from build123d import *

# Parameters (mm, degrees)
BOSS_EXTRUDE1_DEPTH = 24
SKETCH3_R           = 1.9
SKETCH3_R_2         = 0.9
BOSS_EXTRUDE2_DEPTH = 1
SKETCH4_R           = 1.15
CUT_EXTRUDE2_DEPTH  = 4
CUT_EXTRUDE3_DEPTH  = 30


with BuildPart() as part:
    # Sketch1 → Boss-Extrude1 (new body)
    with BuildSketch(Plane(origin=(0, 0, 0), x_dir=(1, 0, 0), z_dir=(0, 1, 0))):
        Polygon((0.758759529, 5.315), (5, 5.315), (5, -7.215), (1.398203198, -7.215), (-1.03, -7.215), (-1.03, -1.785), (4, -1.785), (4, -0.115), (-1.03, -0.115), (-1.03, 5.315), align=None)
    extrude(amount=BOSS_EXTRUDE1_DEPTH)

    # Sketch3 → Boss-Extrude2 (add)
    with BuildSketch(Plane(origin=(5, 0, 0), x_dir=(0, 0, -1), z_dir=(1, 0, 0))):
        with Locations((2.815, 19)):
            Circle(SKETCH3_R)
        with Locations((2.815, 19)):
            Circle(SKETCH3_R_2, mode=Mode.SUBTRACT)
        with Locations((2.815, 5)):
            Circle(SKETCH3_R)
        with Locations((2.815, 5)):
            Circle(SKETCH3_R_2, mode=Mode.SUBTRACT)
    extrude(amount=BOSS_EXTRUDE2_DEPTH)

    # Sketch4 → Cut-Extrude2 (cut)
    with BuildSketch(Plane(origin=(5, 0, 0), x_dir=(0, 0, -1), z_dir=(1, 0, 0))):
        with Locations((2.815, 19)):
            Circle(SKETCH4_R)
        with Locations((2.815, 5)):
            Circle(SKETCH4_R)
    extrude(amount=-CUT_EXTRUDE2_DEPTH, mode=Mode.SUBTRACT)

    # Sketch6 → Cut-Extrude3 (cut)
    with BuildSketch(Plane(origin=(0, 24, 0), x_dir=(1, 0, 0), z_dir=(0, 1, 0))):
        Polygon((-1.03, -0.115), (4, -0.115), (-1.03, 1.385), align=None)
        Polygon((4, -1.785), (-1.03, -1.785), (-1.03, -3.285), align=None)
    extrude(amount=-CUT_EXTRUDE3_DEPTH, mode=Mode.SUBTRACT)


solid = part.part
For this review, take the finished solid that the model builds, in its own axes (mm). A direction names the side the tool comes from. Give positions to 0.01 mm unless a question says otherwise; leave off trailing zeros. Loops run counter-clockwise (first coordinate to the right, second up) from the corner with the lowest first, then second, coordinate; pieces in that order, holes last.
Item 1: For line 1 along X through (y, z) = (18.5, -2); line 2 along Z through (x, y) = (3, 19.5) (3 decimals); line 3 along Y through (x, z) = (4.5, -3.75), list the stretches that pass through material, from the lowest coordinate up.
Item 2: Take a section at B-B, the plane x = 3.25. State the section outline as (y, z) points (3 decimals), and give its area (3 significant figures).
Item 3: Take a section at C-C, the plane z = -2.25. State the section outline as (x, y) points.
Item 4: Tool access review of faces 1 (the cylindrical face through (5.493, 20.884, -2.568)), 2 (the cylindrical face through (3.03, 6.14, -2.67)), 3 (the flat face through (2, 12, -5.315)), 4 (the flat face through (1.45, 12.168, 2.545)): name each direction out of +Z, -Z, +X, -X, +Y, -Y from which nothing blocks a thin tool from reaching the whole face with its end or side.
Item 5: Take a section at A-A, the plane y = 5. State the section outline as (x, z) points (3 decimals), and give its area (3 significant figures).
Item 6: Take a section at D-D, the plane x = 0.5. State the section outline as (y, z) points (3 decimals).
Item 7: Insertion check: pin 1 (1.5 mm diameter, centred on y = 14, z = -3.5, fed in from +X); pin 2 (1.6 mm diameter, centred on y = 19, z = -2.815, fed in from +X). Each pin has a flat end and moves straight along its axis. Give the tip position at first contact, or say it passes through.
Item 8: Draft analysis for pull direction Z (two halves, no side actions). For faces 5 (the cylindrical face through (5.493, 19.892, -2.698)), 6 (the cylindrical face through (5.49, 6.6, -3.84)), 7 (the flat face through (-1.03, 12, -3)), state which applies: +Z half, -Z half, draft (parallel to the pull), parting line (faces both ways), or undercut.
Calculated:
1. line 1: x = -1.03 to 1, 5 to 6
1. line 2: z = -5.315 to -3.851, -1.779 to -0.183, 2.083 to 7.215
1. line 3: y = 0 to 4.33, 5.67 to 18.33, 19.67 to 24
2. outline: (0, -5.315) - (24, -5.315) - (24, -0.109) - (0, -0.109) - close; (0, 2.009) - (24, 2.009) - (24, 7.215) - (0, 7.215) - close; hole circle Ø2.3 at (5, -2.815); hole circle Ø2.3 at (19, -2.815)
2. area: 242 mm2
3. outline: (-1.03, 0) - (5, 0) - (5, 3.19) - (6, 3.19) - (6, 4.3) - (5, 4.3) - (5, 4) - (1, 4) - (1, 6) - (5, 6) - (5, 5.7) - (6, 5.7) - (6, 6.81) - (5, 6.81) - (5, 17.19) - (6, 17.19) - (6, 18.3) - (5, 18.3) - (5, 18) - (1, 18) - (1, 20) - (5, 20) - (5, 19.7) - (6, 19.7) - (6, 20.81) - (5, 20.81) - (5, 24) - (-1.03, 24) - close
4. face 1: +X
4. face 2: none
4. face 3: -Z, +X, -X, +Y, -Y
4. face 4: -X, +Y, -Y
5. outline: (-1.03, -5.315) - (5, -5.315) - (5, -4.715) - (6, -4.715) - (6, -3.715) - (5, -3.715) - (5, -3.965) - (1, -3.965) - (1, -1.665) - (5, -1.665) - (5, -1.915) - (6, -1.915) - (6, -0.915) - (5, -0.915) - (5, 7.215) - (-1.03, 7.215) - (-1.03, 3.285) - (4, 1.785) - (4, 0.115) - (-1.03, -1.385) - close
5. area: 52.4 mm2
6. outline: (0, -5.315) - (24, -5.315) - (24, -0.929) - (0, -0.929) - close; (0, 2.829) - (24, 2.829) - (24, 7.215) - (0, 7.215) - close
7. pin 1: stops at x = 5
7. pin 2: stops at x = 1
8. face 5: undercut
8. face 6: parting line
8. face 7: draft
